Autodesk Inventor part; units mm, degrees
ref_plane "axle_XY" through (0, 0, 0) normal (0, 0, -1) x (1, 0, 0)
ref_plane "axle_YZ" through (0, 0, 0) normal (1, 0, 0) x (0, -1, 0)
ref_plane "axle_ZX" through (0, 0, 0) normal (0, -1, 0) x (0, 0, -1)
sketch "Sketch_2" plane through (0, 0, 0) normal (1, 0, 0) x (0, 1, 0)
  line L0 (0, -52.324) -> (0, 6.096)
  line L1 (0, 6.096) -> (7.112, 6.096)
  line L2 (7.112, 6.096) -> (8.5344, 5.2748)
  line L3 (8.5344, 5.2748) -> (8.5344, 0.8212)
  line L4 (8.5344, 0.8212) -> (7.112, 0)
  line L5 (7.112, 0) -> (4.7625, 0)
  line L6 (4.7625, 0) -> (4.7625, -51.3779)
  line L7 (4.7625, -51.3779) -> (3.8163, -52.324)
  line L8 (3.8163, -52.324) -> (0, -52.324)
  line L9 (0, -52.324) -> (0, 6.096)
revolve "Revolution1" add sketch "Sketch_2" angle 360 about axis through (0, 0, -52.324) along (0, 0, -1)
thread "Thread1"
sketch "Sketch_5" plane through (0, 0, 0) normal (0, 0, 1) x (1, 0, 0)
  circle A0 centre (0, 0) radius 12.7
  line L0 (-7.112, -4.1061) -> (0, -8.2122)
  line L1 (0, -8.2122) -> (7.112, -4.1061)
  line L2 (7.112, -4.1061) -> (7.112, 4.1061)
  line L3 (7.112, 4.1061) -> (0, 8.2122)
  line L4 (0, 8.2122) -> (-7.112, 4.1061)
  line L5 (-7.112, 4.1061) -> (-7.112, -4.1061)
extrude "Extrusion1" cut sketch "Sketch_5" along normal blind 25.4
ref_plane "axle_XY" through (0, 0, 0) normal (0, 0, -1) x (1, 0, 0)
ref_plane "axle_YZ" through (0, 0, 0) normal (1, 0, 0) x (0, -1, 0)
ref_plane "axle_ZX" through (0, 0, 0) normal (0, -1, 0) x (0, 0, -1)
properties part number "2.05456-A"
Source: CAD feature listing. Evaluate the final solid. Frame: model axes, mm. A direction names the side the tool comes from. Give positions to 0.01 mm unless a question says otherwise; leave off trailing zeros. Loops run counter-clockwise (first coordinate to the right, second up) from the corner with the lowest first, then second, coordinate; pieces in that order, holes last. Notation, with made-up numbers: (29, 28.25) -> (61, 28.25) arc R22 ccw to (61, 56.25) -> close; hole circle Ø10 at (-11, 68). An arc over 180 degrees is marked (long way). Use a Markdown table: item, result. Add a question column.
(1) Access query for faces 1 (the face through (-5, 1, 0)), 2 (the face through (3.61, 6.13, 3.01)). Directions: +Z, -Z, +X, -X, +Y, -Y. A direction counts if a zero-diameter tool reaches every point of the face in a straight line with its end or side. Return the directions, or none.
(2) Ray query, line 1 (Z direction, x = -1.25, y = 6.5); line 2 (X direction, y = -4, z = -46); line 3 (Z direction, x = -0.5, y = -4.5). Return the intervals inside material, ascending.
(3) Section query A-A (z = -34). Output: boundary loops of the cut face in (x, y) (1 decimal).
(4) First-contact query: pin 1 Ø5 at (x, z) = (-2.5, -4.5) entering from -Y; pin 2 Ø8 at (x, z) = (-3.5, -36) entering from +Y; pin 3 Ø4 at (x, y) = (-4, -5) entering from -Z. Flat tips, straight axial feed; report the tip coordinate or a pass-through.
Checked values:
| question | item | result |
|---|---|---|
| 1 | face 1 | -Z |
| 1 | face 2 | +Z, -Z, +X, +Y |
| 2 | line 1 | 0 to 6.1 |
| 2 | line 2 | -2.58 to 2.58 |
| 2 | line 3 | -51.61 to 6.1 |
| 3 | outline | circle Ø9.5 at (0, 0) |
| 4 | pin 1 | y = -4.76 |
| 4 | pin 2 | y = 4.76 |
| 4 | pin 3 | z = -51.74 |
